Design review of the part built by this model. Coordinates are the model's own, in mm. A direction names the side the tool comes from. Coordinates: 2 decimals unless noted, no trailing zeros. Write each loop counter-clockwise with the first axis right and the second up, starting at its lowest first coordinate (ties: lowest second). Pieces come first, ordered by that corner, then holes. Notation, with made-up numbers: (54.5, -17) -> (66.5, -17) arc R34 cw to (66.5, 17) -> close; hole circle Ø11 at (44, 54.5). An arc over 180 degrees is marked (long way). Return JSON: item names as keys, results as strings. Group by question number.
from build123d import *

# Parameters (mm, degrees)
BOSS_EXTRUDE1_DEPTH = 20
CUT_EXTRUDE1_DEPTH  = 20
BOSS_EXTRUDE3_DEPTH = 20
SKETCH6_R           = 7.5
CUT_EXTRUDE3_DEPTH  = 10
SHELL2_START        = 5
SHELL2_DEPTH        = 10


# Read off the part's stored shape, not the designer's step: Shell2
with BuildPart() as part:
    # Sketch2 → Boss-Extrude1 (new body)
    with BuildSketch(Plane.XY):
        Polygon((-219.402985075, 0), (-619.402985075, 300), (580.597014925, 300), (180.597014925, 0), align=None)
    extrude(amount=BOSS_EXTRUDE1_DEPTH)

    # Sketch3 → Cut-Extrude1 (cut)
    with BuildSketch(Plane.XY.offset(20)):
        Polygon((-529.402985075, 270), (-209.402985075, 30), (170.597014925, 30), (490.597014925, 270), align=None)
    extrude(amount=-CUT_EXTRUDE1_DEPTH, mode=Mode.SUBTRACT)

    # Sketch4 → Boss-Extrude3 (add)
    with BuildSketch(Plane.XY.offset(20)):
        Polygon((-219.402985075, 270), (-219.402985075, 37.5), (-219.402985075, 30), (-189.402985075, 30), (-189.402985075, 251.618524964), (-197.626477217, 257.431891774), (-189.402985075, 269.064707185), (-189.402985075, 270), align=None)
        Polygon((-180.308988395, 281.928923858), (-189.402985075, 269.064707185), (-189.402985075, 251.618524964), (141.766056114, 17.507872327), (150.597014925, 30), (150.597014925, 48.004218454), align=None)
        Polygon((-189.402985075, 251.618524964), (-189.402985075, 269.064707185), (-197.626477217, 257.431891774), align=None)
        Polygon((158.892990534, 42.497071205), (150.597014925, 48.004218454), (150.597014925, 30), align=None)
        Polygon((150.597014925, 270), (150.597014925, 48.004218454), (158.892990534, 42.497071205), (150.597014925, 30), (180.597014925, 30), (180.597014925, 37.5), (180.597014925, 270), align=None)
    extrude(amount=-BOSS_EXTRUDE3_DEPTH)

    # Sketch6 → Cut-Extrude3 (cut)
    with BuildSketch(Plane.XY.offset(20)):
        with Locations((-204.402985075, 285)):
            Circle(SKETCH6_R)
        with Locations((-204.402985075, 15)):
            Circle(SKETCH6_R)
        with Locations((165.597014925, 15)):
            Circle(SKETCH6_R)
        with Locations((165.597014925, 285)):
            Circle(SKETCH6_R)
        with Locations((525.597014925, 285)):
            Circle(SKETCH6_R)
        with Locations((-562.046220464, 285)):
            Circle(SKETCH6_R)
    extrude(amount=-CUT_EXTRUDE3_DEPTH, mode=Mode.SUBTRACT)

    # Shell2 outline → Shell2 (cut)
    with BuildSketch(Plane.XY.offset(SHELL2_START)):
        with BuildLine():
            ThreePointArc((-554.546220464, 295), (-562.046220464, 272.5), (-569.546220464, 295))
            Line((-569.546220464, 295), (-604.402985075, 295))
            Line((-604.402985075, 295), (-217.736318408, 5))
            Line((-217.736318408, 5), (-211.902985075, 5))
            ThreePointArc((-211.902985075, 5), (-204.402985075, 27.5), (-196.902985075, 5))
            Line((-196.902985075, 5), (158.097014925, 5))
            ThreePointArc((158.097014925, 5), (165.597014925, 27.5), (173.097014925, 5))
            Line((173.097014925, 5), (178.930348259, 5))
            Line((178.930348259, 5), (565.597014925, 295))
            Line((565.597014925, 295), (533.097014925, 295))
            ThreePointArc((533.097014925, 295), (525.597014925, 272.5), (518.097014925, 295))
            Line((518.097014925, 295), (173.097014925, 295))
            ThreePointArc((173.097014925, 295), (165.597014925, 272.5), (158.097014925, 295))
            Line((158.097014925, 295), (-196.902985075, 295))
            ThreePointArc((-196.902985075, 295), (-204.402985075, 272.5), (-211.902985075, 295))
            Line((-211.902985075, 295), (-554.546220464, 295))
        make_face()
        Polygon((-544.402985075, 275), (-214.402985075, 275), (-214.402985075, 27.5), align=None, mode=Mode.SUBTRACT)
        Polygon((-194.402985075, 275), (155.597014925, 275), (155.597014925, 38.346418141), (-179.112397852, 274.95983704), (-190.657390399, 258.628482317), (139.829580663, 25), (-194.402985075, 25), align=None, mode=Mode.SUBTRACT)
        Polygon((175.597014925, 275), (505.597014925, 275), (175.597014925, 27.5), align=None, mode=Mode.SUBTRACT)
    extrude(amount=SHELL2_DEPTH, mode=Mode.SUBTRACT)


solid = part.part
Q1. For faces 3 (the flat face through (338, 270, 10)), 4 (the cylindrical face through (165.16, 27.492, 9.93)), 5 (the flat face through (383.4, 152.1, 9.9)), list the 3-axis set-ups (+Z, -Z, +X, -X, +Y, -Y) from which the entire face can be reached by the end or side of a thin tool; tool diameter is ignored.
Q2. We need section B-B on x = 236. Write out the cut boundary in (y, z).
Q3. For P1, Ø8, axis at y = 154.5, z = 10.5, coming from the -X side; P2, Ø12, axis at x = 525.6, y = 285, coming from the +Z side; P3, Ø11, axis at x = 543, z = 8.5, coming from the -Y side, all flat-tipped, find the tip position at first contact; note any pin that passes through.
Q4. Wall thickness on L1, parallel to Z at x = -48.5, y = 170; L2, parallel to X at y = 285, z = 15.75; L3, parallel to Y at x = 169, z = 17.75: over which ranges is each line inside the solid? List them lowest first.
Q5. The part is to be moulded in two halves that separate along Z. For faces 1 (the flat face through (-413.776, 152.03, 9.93)), 2 (the flat face through (-28, 300, 10)), say which applies: +Z half, -Z half, draft (parallel to the pull), parting line (faces both ways), or undercut.
Q6. We need section A-A on x = 5.5. Write out the cut boundary in (y, z).
Q7. We need section C-C on y = 225. State how many separate pieces and enclosed holes the cut face has, plus the area to 3 significant figures.
Findings below:
{
 "1": {"face 3": "+Z, -Z", "face 4": "none", "face 5": "+Z, -Z, +X, -Y"},
 "2": {"outline": "(41.55, 0) -> (79.05, 0) -> (79.05, 20) -> (41.55, 20) -> close; (270, 0) -> (300, 0) -> (300, 20) -> (270, 20) -> close; hole (47.8, 5) -> (72.8, 5) -> (72.8, 15) -> (47.8, 15) -> close; hole (275, 5) -> (295, 5) -> (295, 15) -> (275, 15) -> close"},
 "3": {"P1": "stops at x = -430.74", "P2": "stops at z = 10", "P3": "stops at y = 267.68"},
 "4": {"L1": "z = 0 to 5, 15 to 20", "L2": "x = -599.4 to -569.55, -554.55 to -211.9, -196.9 to 158.1, 173.1 to 518.1, 533.1 to 560.6", "L3": "y = 0 to 8.32, 21.68 to 278.32, 291.68 to 300"},
 "5": {"face 1": "undercut", "face 2": "draft"},
 "6": {"outline": "(0, 0) -> (30, 0) -> (30, 20) -> (0, 20) -> close; (113.84, 0) -> (150.58, 0) -> (150.58, 20) -> (113.84, 20) -> close; (270, 0) -> (300, 0) -> (300, 20) -> (270, 20) -> close; hole (5, 5) -> (25, 5) -> (25, 15) -> (5, 15) -> close; hole (119.96, 5) -> (144.45, 5) -> (144.45, 15) -> (119.96, 15) -> close; hole (275, 5) -> (295, 5) -> (295, 15) -> (275, 15) -> close"},
 "7": {"separate pieces": "5", "enclosed holes": "5", "area": "2,830 mm^2"}
}
